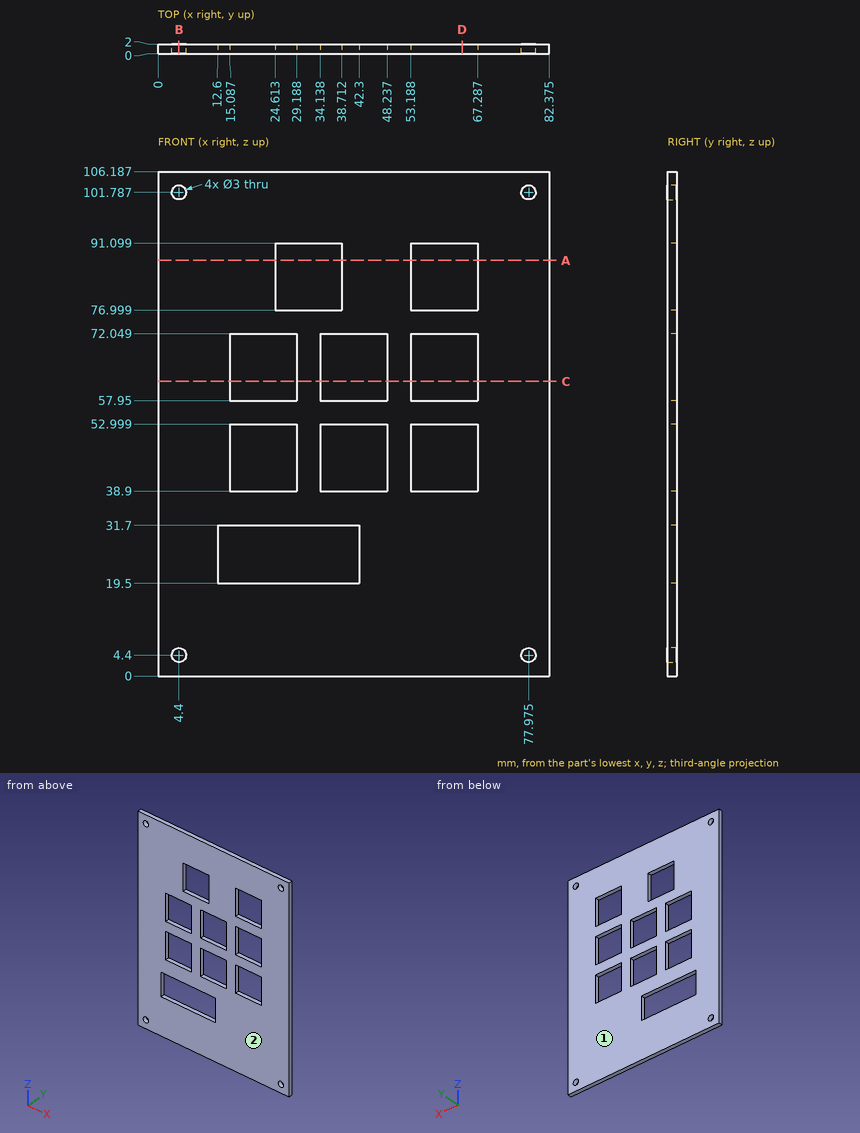
Verification items for this drawing (mm, ordinates from the low corner). Give positions to 0.01 mm unless a question says otherwise; leave off trailing zeros. Loops run counter-clockwise (first coordinate to the right, second up) from the corner with the lowest first, then second, coordinate; pieces in that order, holes last.
1. Material ranges on probe 1 along Z at (x, y) = (29, 1.45); probe 2 along Z at (x, y) = (34, 0.9); probe 3 along Z at (x, y) = (47.5, 1.35), recorded low to high.
Derived:
probe 1: z = 0 to 19.5, 31.7 to 38.9, 53 to 57.95, 72.05 to 77, 91.1 to 106.19
probe 2: z = 0 to 19.5, 31.7 to 77, 91.1 to 106.19
probe 3: z = 0 to 38.9, 53 to 57.95, 72.05 to 106.19
2. Cross-section at A-A on z = 87.5. Record the cut outline in (x, y) (1 decimal).
Derived:
outline: (0, 0) - (24.6, 0) - (24.6, 2) - (0, 2) - close; (38.7, 0) - (53.2, 0) - (53.2, 2) - (38.7, 2) - close; (67.3, 0) - (82.4, 0) - (82.4, 2) - (67.3, 2) - close
3. Cross-section at D-D on x = 64. Record the cut outline in (y, z).
Derived:
outline: (0, 0) - (2, 0) - (2, 38.9) - (0, 38.9) - close; (0, 53) - (2, 53) - (2, 57.95) - (0, 57.95) - close; (0, 72.05) - (2, 72.05) - (2, 77) - (0, 77) - close; (0, 91.1) - (2, 91.1) - (2, 106.19) - (0, 106.19) - close
4. Release check for a two-part mould opening along Y. For the marked faces 1 and 2 record: +Y half, -Y half, draft (parallel to the pull), parting line (faces both ways), or undercut.
Derived:
face 1: +Y half
face 2: -Y half
5. Cross-section at B-B on x = 4.4. Record the cut outline in (y, z).
Derived:
outline: (0, 0) - (2, 0) - (2, 2.9) - (0, 2.9) - close; (0, 5.9) - (2, 5.9) - (2, 100.29) - (0, 100.29) - close; (0, 103.29) - (2, 103.29) - (2, 106.19) - (0, 106.19) - close
6. Cross-section at C-C on z = 62. Record the cut outline in (x, y) (1 decimal).
Derived:
outline: (0, 0) - (15.1, 0) - (15.1, 2) - (0, 2) - close; (29.2, 0) - (34.1, 0) - (34.1, 2) - (29.2, 2) - close; (48.2, 0) - (53.2, 0) - (53.2, 2) - (48.2, 2) - close; (67.3, 0) - (82.4, 0) - (82.4, 2) - (67.3, 2) - close
